Model file for the job. Use its own axes, mm. A direction names the side the tool comes from. Coordinates: 2 decimals unless noted, no trailing zeros. Order: outer loops, then holes, each group sorted by start corner. A loop starts at its lowest first (then second) coordinate and runs counter-clockwise, first axis right, second up. Notation, with made-up numbers: M -35,-37.75 L 21,-37.75 A19 ccw 21,-10.75 Z; hole C 10.5,-1 d3. An arc over 180 degrees is marked long. Return JSON: item names as keys, results as strings.
```python
from build123d import *

# Parameters (mm, degrees)
ESQUISSE1_W        = 19.9
ESQUISSE1_H        = 10.4
BOSS_EXTRU_1_DEPTH = 3.25
D_GAGEMENT_M2_51_D = 2.7
ESQUISSE4_W        = 0.4
ESQUISSE4_H        = 3.1
BOSS_EXTRU_2_DEPTH = 3.5
ESQUISSE5_W        = 1.8
ESQUISSE5_H        = 3.9
BOSS_EXTRU_3_DEPTH = 1.5
BOSS_EXTRU_4_DEPTH = 2


with BuildPart() as part:
    # Esquisse1 → Boss.-Extru.1 (new, symmetric)
    with BuildSketch(Plane.XY):
        Rectangle(ESQUISSE1_W, ESQUISSE1_H)
    extrude(amount=BOSS_EXTRU_1_DEPTH, both=True)

    # Dégagement M2.51 (through all)
    with Locations(Plane.XY.offset(3.25)):
        with Locations((-4.75, -2.2), (4.75, -2.2)):
            Hole(D_GAGEMENT_M2_51_D / 2)

    # Esquisse4 → Boss.-Extru.2 (add)
    with BuildSketch(Plane.XZ.offset(5.2)):
        with Locations((0.5, 0)):
            Rectangle(ESQUISSE4_W, ESQUISSE4_H)
        with Locations((8, 0)):
            Rectangle(ESQUISSE4_W, ESQUISSE4_H)
        with Locations((-8, 0)):
            Rectangle(ESQUISSE4_W, ESQUISSE4_H)
    extrude(amount=BOSS_EXTRU_2_DEPTH)

    # Esquisse5 → Boss.-Extru.3 (add)
    with BuildSketch(Plane(origin=(0, 5.2, 0), x_dir=(1, 0, 0), z_dir=(0, 1, 0))):
        with Locations((-3.35, 0)):
            Rectangle(ESQUISSE5_W, ESQUISSE5_H)
    extrude(amount=BOSS_EXTRU_3_DEPTH)

    # Esquisse6 → Boss.-Extru.4 (add, symmetric)
    with BuildSketch(Plane.XY):
        Polygon((-6.7, 5.2), (-6.7, 6.2), (21.05, 6.2), (21.05, 6.45), (-6.95, 6.45), (-6.95, 5.2), align=None)
    extrude(amount=BOSS_EXTRU_4_DEPTH, both=True)


solid = part.part
```
Item 1: Pull direction X, two halves, no side cores. Call faces 5 (the flat face through (-3, 6.7, 0)), 6 (the flat face through (-4.25, 6, 0)), 7 (the flat face through (-8.2, -7, 0)): +X half, -X half, draft (parallel to the pull), parting line (faces both ways), or undercut.
Check result:
{"face 5": "draft", "face 6": "undercut", "face 7": "-X half"}
Item 2: 3-axis set-ups, long thin cutter, end or side, ignore diameter. For faces 1 (the flat face through (9.95, 0, 0)), 2 (the flat face through (0.7, -7, 0)), 3 (the flat face through (-6.7, 6, 0)), 4 (the flat face through (-2.45, 6, 0)): which of +Z, -Z, +X, -X, +Y, -Y reach the whole face in a straight line?
Check result:
{"face 1": "+Z, -Z, +X, -Y", "face 2": "+Z, -Z, -Y", "face 3": "+Z, -Z", "face 4": "+Z, -Z, +X"}
Item 3: Saw through at D-D (y = -0.25). Write the cut outline in (x, z).
Check result:
{"outline": "M -9.95,-3.25 L 9.95,-3.25 L 9.95,3.25 L -9.95,3.25 Z"}
Item 4: Wall check: line 1 (Y direction, x = 4.75, z = -1.5); line 2 (Y direction, x = -6.5, z = 1.5); line 3 (Y direction, x = -4.75, z = 2.25). Give the ranges that are in metal, low to high.
Check result:
{"line 1": "y = -5.2 to -3.55, -0.85 to 5.2, 6.2 to 6.45", "line 2": "y = -5.2 to 5.2, 6.2 to 6.45", "line 3": "y = -5.2 to -3.55, -0.85 to 5.2"}
Item 5: Saw through at B-B (y = -2.2). Write the cut outline in (x, z), and give its area (4 significant figures).
Check result:
{"outline": "M -9.95,-3.25 L -6.1,-3.25 L -6.1,3.25 L -9.95,3.25 Z; M -3.4,-3.25 L 3.4,-3.25 L 3.4,3.25 L -3.4,3.25 Z; M 6.1,-3.25 L 9.95,-3.25 L 9.95,3.25 L 6.1,3.25 Z", "area": "94.25 mm2"}
Item 6: Saw through at C-C (z = 0.75). Count the separate pieces of the cut face and the enclosed holes in it, and give its area (3 significant figures).
Check result:
{"separate pieces": "1", "enclosed holes": "3", "area": "209 mm2"}
Item 7: Drop flat-ended pins along their axis: pin 1 Ø1 at (y, z) = (-2.5, 1.5) entering from +X; pin 2 Ø1.6 at (x, y) = (4.75, -2.2) entering from -Z; pin 3 Ø0.9 at (y, z) = (-7.5, 0) entering from -X; pin 4 Ø1.2 at (x, z) = (12, 0) entering from +Y. Give the stop position or say it passes through.
Check result:
{"pin 1": "stops at x = 9.95", "pin 2": "passes through", "pin 3": "stops at x = -8.2", "pin 4": "stops at y = 6.45"}
Item 8: Saw through at A-A (x = -4.75). Write the cut outline in (y, z), and give its area (4 significant figures).
Check result:
{"outline": "M -5.2,-3.25 L -3.55,-3.25 L -3.55,3.25 L -5.2,3.25 Z; M -0.85,-3.25 L 5.2,-3.25 L 5.2,3.25 L -0.85,3.25 Z; M 6.2,-2 L 6.45,-2 L 6.45,2 L 6.2,2 Z", "area": "51.05 mm2"}
